from build123d import *

# Parameters (mm, degrees)
DODANIE_WYCI_GNI_CIE1_DEPTH = 1
SZKIC2_R                    = 3.15
WYTNIJ_WYCI_GNI_CIE1_DEPTH  = 1


with BuildPart() as part:
    # Szkic1 → Dodanie-wyciągnięcie1 (new body)
    with BuildSketch(Plane.XY):
        with BuildLine():
            Line((-12.5, -6), (-12.5, -16))
            Line((-12.5, -16), (12.5, -16))
            Line((12.5, -16), (12.5, -6))
            Line((12.5, -6), (7.91, -6))
            ThreePointArc((7.91, -6), (6.495786438, -5.414213562), (5.91, -4))
            Line((5.91, -4), (5.91, 15.65))
            Line((5.91, 15.65), (-5.85, 15.65))
            Line((-5.85, 15.65), (-5.85, -4))
            ThreePointArc((-5.85, -4), (-6.435786438, -5.414213562), (-7.85, -6))
            Line((-7.85, -6), (-12.5, -6))
        make_face()
    extrude(amount=DODANIE_WYCI_GNI_CIE1_DEPTH)

    # Szkic2 → Wytnij-wyciągnięcie1 (cut)
    with BuildSketch(Plane.XY.offset(1)):
        with Locations((0.03, 10.16)):
            Circle(SZKIC2_R)
    extrude(amount=-WYTNIJ_WYCI_GNI_CIE1_DEPTH, mode=Mode.SUBTRACT)


solid = part.part
Could you check a few things on this model? Use its own coordinates, in mm. A direction names the side the tool comes from. Coordinates: 2 decimals unless noted, no trailing zeros. Order: outer loops, then holes, each group sorted by start corner. A loop starts at its lowest first (then second) coordinate and runs counter-clockwise, first axis right, second up.
Q1. Suppose I cut it at A-A on y = 10.16. Please give me the cut outline in (x, z).
Q2. Will these pins go through, and if not, where does the flat tip stop? pin 1 (0.5 mm diameter, centred on y = 5.5, z = 0.5, fed in from -X); pin 2 (5 mm diameter, centred on x = 0.03, y = 10.16, fed in from -Z); pin 3 (0.5 mm diameter, centred on y = 10, z = 0.5, fed in from +X).
Q3. Thinking about a two-plate mould opening in Y: for faces 1 (the cylindrical face through (-0.38, 13.283, 0.507)), 2 (the flat face through (-5.85, 6, 0.5)), 3 (the flat face through (10.2, -6, 0.5)), which applies, released by +Y, released by -Y, zero draft, split by the parting line, or undercut?
Q4. Please list where these lines run through material, in increasing order: L1, parallel to Y at x = 0.03, z = 0.6; L2, parallel to Y at x = -9.25, z = 0.35; L3, parallel to X at y = 14.5, z = 0.5.
Q5. Which directions (+Z, -Z, +X, -X, +Y, -Y) give clear straight access to the entire face, cutting with the end or side of a thin tool? Please do faces 4 (the flat face through (-10.1, -6, 0.5)), 5 (the flat face through (5.91, 5.7, 0.5)), 6 (the flat face through (0.1, 15.65, 0.5)).
Q6. Suppose I cut it at B-B on x = 0.03. Please give me the cut outline in (y, z).
Q7. Suppose I cut it at C-C on z = 0.7. Please give me the cut outline in (x, y), and give its area (3 significant figures).
Q8. Suppose I cut it at D-D on y = 6.5. Please give me the cut outline in (x, z).
Answer:
1. outline: (-5.85, 0) - (-3.12, 0) - (-3.12, 1) - (-5.85, 1) - close; (3.18, 0) - (5.91, 0) - (5.91, 1) - (3.18, 1) - close
2. pin 1: stops at x = -5.85
2. pin 2: passes through
2. pin 3: stops at x = 5.91
3. face 1: undercut
3. face 2: zero draft
3. face 3: released by +Y
4. L1: y = -16 to 7.01, 13.31 to 15.65
4. L2: y = -16 to -6
4. L3: x = -5.85 to 5.91
5. face 4: +Z, -Z, -X, +Y
5. face 5: +Z, -Z, +X, +Y
5. face 6: +Z, -Z, +X, -X, +Y
6. outline: (-16, 0) - (7.01, 0) - (7.01, 1) - (-16, 1) - close; (13.31, 0) - (15.65, 0) - (15.65, 1) - (13.31, 1) - close
7. outline: (-12.5, -16) - (12.5, -16) - (12.5, -6) - (7.91, -6) arc R2 cw to (5.91, -4) - (5.91, 15.65) - (-5.85, 15.65) - (-5.85, -4) arc R2 cw to (-7.85, -6) - (-12.5, -6) - close; hole circle Ø6.3 at (0.03, 10.16)
7. area: 475 mm2
8. outline: (-5.85, 0) - (5.91, 0) - (5.91, 1) - (-5.85, 1) - close
